Model file for the job. Use its own axes, mm. Coordinates: 2 decimals unless noted, no trailing zeros. Order: outer loops, then holes, each group sorted by start corner. A loop starts at its lowest first (then second) coordinate and runs counter-clockwise, first axis right, second up. Notation, with made-up numbers: M -23,73.5 L 21,73.5 A29 ccw 21,112.5 Z; hole C -14.75,20 d3. An arc over 180 degrees is marked long. Return JSON: item names as keys, results as strings.
Autodesk Inventor part; units mm, degrees
ref_plane "YZ Plane" through (0, 0, 0) normal (1, 0, 0) x (0, 1, 0)
ref_plane "XZ Plane" through (0, 0, 0) normal (0, 1, 0) x (-1, 0, 0)
ref_plane "XY Plane" through (0, 0, 0) normal (0, 0, 1) x (1, 0, 0)
sketch "Sketch1" plane through (0, 0, 0) normal (0, 0, 1) x (1, 0, 0)
  line L0 (0, 0) -> (355.6, 0)
  line L1 (355.6, 0) -> (355.6, 152.4)
  line L2 (355.6, 152.4) -> (0, 152.4)
  line L3 (0, 152.4) -> (0, 0)
  dimension "d0" = 152.4
  dimension "d1" = 355.6
extrude "Extrusion1" add sketch "Sketch1" along normal blind 3.175
sketch "Sketch2" plane through (0, 0, 3.175) normal (0, 0, 1) x (1, 0, 0)
  line L0 (50.8, 50.8) -> (105.918, 50.8)
  line L1 (105.918, 50.8) -> (105.918, 86.36)
  line L2 (105.918, 86.36) -> (50.8, 86.36)
  line L3 (50.8, 86.36) -> (50.8, 50.8)
  line L4 (0, 152.4) -> (0, 0)
  line L5 (0, 0) -> (355.6, 0)
  dimension "d4" = 55.118
  dimension "d5" = 35.56
  dimension "d6" = 50.8
  dimension "d7" = 50.8
extrude "Extrusion2" cut sketch "Sketch2" against normal blind 3.175
sketch "Sketch3" plane through (0, 0, 3.175) normal (0, 0, 1) x (1, 0, 0)
  circle A0 centre (199.136, 69.85) radius 12.7
  circle A1 centre (286.5628, 82.804) radius 12.7
  line L0 (0, 0) -> (355.6, 0)
  line L1 (0, 152.4) -> (0, 0)
  line L2 (355.6, 0) -> (355.6, 152.4)
  dimension "d10" = 25.4
  dimension "d11" = 25.4
  dimension "d12" = 69.85
  dimension "d13" = 82.804
  dimension "d14" = 199.136
  dimension "d15" = 69.0372
extrude "Extrusion3" cut sketch "Sketch3" against normal blind 3.175
sketch "Sketch4" plane through (0, 0, 3.175) normal (0, 0, 1) x (1, 0, 0)
  line L0 (0, 0) -> (355.6, 0)
  line L1 (0, 152.4) -> (0, 0)
  point P0 (40.64, 41.91)
  point P1 (116.84, 41.91)
  point P2 (116.84, 92.71)
  point P3 (40.64, 92.71)
  dimension "d18" = 41.91
  dimension "d19" = 41.91
  dimension "d20" = 92.71
  dimension "d21" = 92.71
  dimension "d22" = 40.64
  dimension "d23" = 116.84
  dimension "d24" = 40.64
  dimension "d25" = 116.84
hole "Hole1" at (40.64, 41.91, 3.175) at (116.84, 41.91, 3.175) at (116.84, 92.71, 3.175) at (40.64, 92.71, 3.175) direction (0, 0, -1) diameter 3.302 end through all
fillet "Fillet1" radius 3.175 4 edges at (50.8, 50.8, 1.5875) (105.918, 86.36, 1.5875) (105.918, 50.8, 1.5875) (50.8, 86.36, 1.5875)
properties part number "LFEV2017_TSI_003"
Item 1: Saw through at A-A (x = 60). Write the cut outline in (y, z) (3 decimals).
Check result:
{"outline": "M 0,0 L 50.8,0 L 50.8,3.175 L 0,3.175 Z; M 86.36,0 L 152.4,0 L 152.4,3.175 L 86.36,3.175 Z"}
Item 2: Saw through at B-B (z = 2.3). Write the cut outline in (x, y) (3 decimals), and give its area (3 significant figures).
Check result:
{"outline": "M 0,0 L 355.6,0 L 355.6,152.4 L 0,152.4 Z; hole C 40.64,41.91 d3.302; hole C 40.64,92.71 d3.302; hole M 50.8,53.975 A3.175 ccw 53.975,50.8 L 102.743,50.8 A3.175 ccw 105.918,53.975 L 105.918,83.185 A3.175 ccw 102.743,86.36 L 53.975,86.36 A3.175 ccw 50.8,83.185 Z; hole C 116.84,41.91 d3.302; hole C 116.84,92.71 d3.302; hole C 199.136,69.85 d25.4; hole C 286.563,82.804 d25.4", "area": "51,200 mm2"}
Item 3: Wall check: line 1 (Y direction, x = 116.84, z = 1.75); line 2 (X direction, y = 92.71, z = 1); line 3 (Y direction, x = 64, z = 0.9). Give the ranges that are in metal, low to high.
Check result:
{"line 1": "y = 0 to 40.26, 43.56 to 91.06, 94.36 to 152.4", "line 2": "x = 0 to 38.99, 42.29 to 115.19, 118.49 to 278.62, 294.51 to 355.6", "line 3": "y = 0 to 50.8, 86.36 to 152.4"}
Item 4: Drop flat-ended pins along their axis: pin 1 Ø4.5 at (x, y) = (40.64, 41.91) entering from -Z; pin 2 Ø2.5 at (x, y) = (40.64, 92.71) entering from +Z. Give the stop position or say it passes through.
Check result:
{"pin 1": "stops at z = 0", "pin 2": "passes through"}
Item 5: Pull direction Y, two halves, no side cores. Call faces 1 (the flat face through (175, 77, 0)), 2 (the cylindrical face through (298.676, 86.619, 1.61)): +Y half, -Y half, draft (parallel to the pull), parting line (faces both ways), or undercut.
Check result:
{"face 1": "draft", "face 2": "undercut"}
Item 6: Saw through at C-C (x = 294). Write the cut outline in (y, z) (3 decimals).
Check result:
{"outline": "M 0,0 L 72.509,0 L 72.509,3.175 L 0,3.175 Z; M 93.099,0 L 152.4,0 L 152.4,3.175 L 93.099,3.175 Z"}
